```python
from build123d import *

# Parameters (mm, degrees)
SKETCH_1_W          = 56.21
SKETCH_1_H          = 40.43
EXTRUDE_1_DEPTH     = 1.5
SKETCH_2_W          = 54.71
SKETCH_2_H          = 1.5
EXTRUDE_2_DEPTH     = 3.5
SKETCH_3_W          = 1.5
SKETCH_3_H          = 8
SKETCH_3_H_2        = 18
EXTRUDE_3_DEPTH     = 3.5
SKETCH_4_W          = 2.2
SKETCH_4_H          = 1.8
EXTRUDE_4_DEPTH     = 3.5
SKETCH_5_W          = 2
SKETCH_5_H          = 1.8
EXTRUDE_5_DEPTH     = 3.5
EXTRUDE_9_DEPTH     = 7.5
SKETCH_9_R          = 0.8
CUT_EXTRUDE_1_DEPTH = 7.5
SKETCH_11_W         = 10
SKETCH_11_H         = 4
CUT_EXTRUDE_2_DEPTH = 7.5
CUT_EXTRUDE_3_DEPTH = 15


with BuildPart() as part:
    # 草图1 → 凸台-拉伸1 (new body)
    with BuildSketch(Plane(origin=(0, 0, 0), x_dir=(1, 0, 0), z_dir=(0, 1, 0))):
        with Locations((-10.770778443, 1.999730539)):
            Rectangle(SKETCH_1_W, SKETCH_1_H)
    extrude(amount=EXTRUDE_1_DEPTH)

    # 草图2 → 凸台-拉伸2 (add)
    with BuildSketch(Plane(origin=(0, 1.5, 0), x_dir=(1, 0, 0), z_dir=(0, 1, 0))):
        Polygon((-37.375778443, 22.214730539), (-38.875778443, 22.214730539), (-38.875778443, -18.215269461), (-37.375778443, -18.215269461), (-37.375778443, -16.715269461), (-37.375778443, 20.714730539), align=None)
        with Locations((-10.020778443, 21.464730539)):
            Rectangle(SKETCH_2_W, SKETCH_2_H)
        with Locations((-10.020778443, -17.465269461)):
            Rectangle(SKETCH_2_W, SKETCH_2_H)
    extrude(amount=EXTRUDE_2_DEPTH)

    # 草图3 → 凸台-拉伸3 (add)
    with BuildSketch(Plane(origin=(0, 1.5, 0), x_dir=(1, 0, 0), z_dir=(0, 1, 0))):
        with Locations((16.584221557, -12.715269461)):
            Rectangle(SKETCH_3_W, SKETCH_3_H)
        with Locations((16.584221557, 11.714730539)):
            Rectangle(SKETCH_3_W, SKETCH_3_H_2)
    extrude(amount=EXTRUDE_3_DEPTH)

    # 草图4 → 凸台-拉伸4 (add)
    with BuildSketch(Plane(origin=(0, 1.5, 0), x_dir=(1, 0, 0), z_dir=(0, 1, 0))):
        with Locations((12.934221557, 19.814730539)):
            Rectangle(SKETCH_4_W, SKETCH_4_H)
        Polygon((15.834221557, 16.714730539), (15.834221557, 20.714730539), (14.034221557, 20.714730539), (14.034221557, 18.914730539), (14.034221557, 16.714730539), align=None)
        Polygon((14.034221557, -16.715269461), (15.834221557, -16.715269461), (15.834221557, -12.715269461), (14.034221557, -12.715269461), (14.034221557, -14.915269461), align=None)
        with Locations((12.934221557, -15.815269461)):
            Rectangle(SKETCH_4_W, SKETCH_4_H)
    extrude(amount=EXTRUDE_4_DEPTH)

    # 草图5 → 凸台-拉伸5 (add)
    with BuildSketch(Plane(origin=(0, 1.5, 0), x_dir=(1, 0, 0), z_dir=(0, 1, 0))):
        with Locations((-36.375778443, 19.814730539)):
            Rectangle(SKETCH_5_W, SKETCH_5_H)
        with Locations((-36.375778443, -15.815269461)):
            Rectangle(SKETCH_5_W, SKETCH_5_H)
    extrude(amount=EXTRUDE_5_DEPTH)

    # 草图8 → 凸台-拉伸9 (add)
    with BuildSketch(Plane(origin=(0, 5, 0), x_dir=(1, 0, 0), z_dir=(0, 1, 0))):
        Polygon((17.334221557, -14.915269461), (14.034221557, -14.915269461), (11.834221557, -14.915269461), (11.834221557, -16.715269461), (-35.375778443, -16.715269461), (-35.375778443, -14.915269461), (-37.375778443, -14.915269461), (-37.375778443, 18.914730539), (-35.375778443, 18.914730539), (-35.375778443, 20.714730539), (11.834221557, 20.714730539), (11.834221557, 18.914730539), (14.034221557, 18.914730539), (17.334221557, 18.914730539), (17.334221557, 22.214730539), (-38.875778443, 22.214730539), (-38.875778443, -18.215269461), (17.334221557, -18.215269461), align=None)
    extrude(amount=EXTRUDE_9_DEPTH)

    # 草图9 → 切除-拉伸1 (cut)
    with BuildSketch(Plane(origin=(0, 12.5, 0), x_dir=(1, 0, 0), z_dir=(0, 1, 0))):
        with Locations(Location((15.684221557, 20.564730539, 0), (0, 0, 270))):
            Circle(SKETCH_9_R)
        with Locations(Location((15.684221557, -16.565269461, 0), (0, 0, 270))):
            Circle(SKETCH_9_R)
        with Locations(Location((-37.225778443, 20.564730539, 0), (0, 0, 270))):
            Circle(SKETCH_9_R)
        with Locations(Location((-37.225778443, -16.565269461, 0), (0, 0, 270))):
            Circle(SKETCH_9_R)
    extrude(amount=-CUT_EXTRUDE_1_DEPTH, mode=Mode.SUBTRACT)

    # 草图11 → 切除-拉伸2 (cut)
    with BuildSketch(Plane(origin=(-37.375778443, 0, 0), x_dir=(0, 0, -1), z_dir=(1, 0, 0))):
        with Locations((6.999730539, 3.5)):
            Rectangle(SKETCH_11_W, SKETCH_11_H)
        with Locations((-3.000269461, 3.5)):
            Rectangle(SKETCH_11_W, SKETCH_11_H)
    extrude(amount=-CUT_EXTRUDE_2_DEPTH, mode=Mode.SUBTRACT)

    # 草图14 → 切除-拉伸3 (cut)
    with BuildSketch(Plane(origin=(0, 12.5, 0), x_dir=(1, 0, 0), z_dir=(0, 1, 0))):
        with BuildLine():
            Line((-38.875778443, 22.214730539), (-38.875778443, 21.130415964))
            ThreePointArc((-38.875778443, 21.130415964), (-38.558190057, 21.897142153), (-37.791463868, 22.214730539))
            Line((-37.791463868, 22.214730539), (-38.875778443, 22.214730539))
        make_face()
        with BuildLine():
            ThreePointArc((-37.791463868, -18.215269461), (-38.558190057, -17.897681075), (-38.875778443, -17.130954886))
            Line((-38.875778443, -17.130954886), (-38.875778443, -18.215269461))
            Line((-38.875778443, -18.215269461), (-37.791463868, -18.215269461))
        make_face()
        with BuildLine():
            ThreePointArc((17.334221557, -17.130954886), (17.016633171, -17.897681075), (16.249906982, -18.215269461))
            Line((16.249906982, -18.215269461), (17.334221557, -18.215269461))
            Line((17.334221557, -18.215269461), (17.334221557, -17.130954886))
        make_face()
        with BuildLine():
            Line((17.334221557, 22.214730539), (16.249906982, 22.214730539))
            ThreePointArc((16.249906982, 22.214730539), (17.016633171, 21.897142153), (17.334221557, 21.130415964))
            Line((17.334221557, 21.130415964), (17.334221557, 22.214730539))
        make_face()
    extrude(amount=-CUT_EXTRUDE_3_DEPTH, mode=Mode.SUBTRACT)


solid = part.part
```
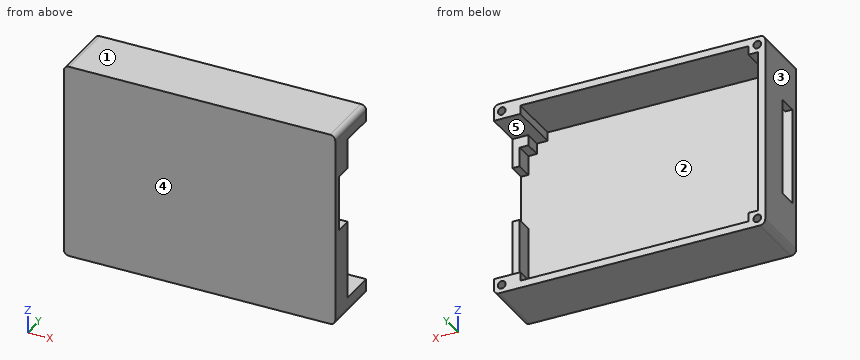
Geometry check sheet. Reference: the model listing, model coordinates, mm. Face numbers are marked on the shaded views. A direction names the side the tool comes from. Give positions to 0.01 mm unless a question says otherwise; leave off trailing zeros. Write each loop counter-clockwise with the first axis right and the second up, starting at its lowest first coordinate (ties: lowest second). Pieces come first, ordered by that corner, then holes. Notation, with made-up numbers: (-1, 75.5) - (46, 75.5) arc R20 cw to (46, 88.5) - close; hole circle Ø3 at (75.5, -15). An arc over 180 degrees is marked (long way). Use a Markdown table: item, result.
Q1. Go/stop test with flat-tipped pins: P1, Ø4, axis at x = -15.5, z = -10.5, coming from the +Y side; P2, Ø1.4, axis at x = 15.68, z = -20.56, coming from the +Y side. Record where each tip stops, or that it passes through.
Computed:
| item | result |
|---|---|
| P1 | stops at y = 1.5 |
| P2 | stops at y = 5 |
Q2. Draft check along X on the marked faces 1, 2 and 3. Enter one of: pulls with the +X half, pulls with the -X half, needs draft (parallel to the pull), parting line crosses it, or undercut.
Computed:
| item | result |
|---|---|
| face 1 | needs draft |
| face 2 | undercut |
| face 3 | pulls with the -X half |
Q3. Section check C-C, the plane x = 5. Enter the section's corners in (y, z), then the cut area to 3 significant figures.
Computed:
| item | result |
|---|---|
| outline | (0, -22.21) - (12.5, -22.21) - (12.5, -20.71) - (1.5, -20.71) - (1.5, 16.72) - (12.5, 16.72) - (12.5, 18.22) - (0, 18.22) - close |
| area | 93.6 mm² |
Q4. Section check D-D, the plane y = 7. Enter the section's corners in (x, z).
Computed:
| item | result |
|---|---|
| outline | (-38.88, -21.13) arc R1.08 ccw to (-37.79, -22.21) - (16.25, -22.21) arc R1.08 ccw to (17.33, -21.13) - (17.33, -18.91) - (11.83, -18.91) - (11.83, -20.71) - (-35.38, -20.71) - (-35.38, -18.91) - (-37.38, -18.91) - (-37.38, 14.92) - (-35.38, 14.92) - (-35.38, 16.72) - (11.83, 16.72) - (11.83, 14.92) - (17.33, 14.92) - (17.33, 17.13) arc R1.08 ccw to (16.25, 18.22) - (-37.79, 18.22) arc R1.08 ccw to (-38.88, 17.13) - close; hole circle Ø1.6 at (-37.23, -20.56); hole circle Ø1.6 at (-37.23, 16.57); hole circle Ø1.6 at (15.68, -20.56); hole circle Ø1.6 at (15.68, 16.57) |
Q5. Section check A-A, the plane z = -9. Enter the section's corners in (x, y).
Computed:
| item | result |
|---|---|
| outline | (-38.88, 0) - (17.33, 0) - (17.33, 5) - (15.83, 5) - (15.83, 1.5) - (-38.88, 1.5) - close; (-38.88, 5.5) - (-37.38, 5.5) - (-37.38, 12.5) - (-38.88, 12.5) - close |
Q6. Thickness scan on L1, parallel to Z at x = -3.5, y = 4.75; L2, parallel to X at y = 3.75, z = 16.5; L3, parallel to X at y = 4.5, z = 12.5. Record the ranges inside material, lowest first. Write a range as [from, to].
Computed:
| item | result |
|---|---|
| L1 | z = [-22.21, -20.71], [16.72, 18.22] |
| L2 | x = [-38.88, -35.38], [11.83, 17.33] |
| L3 | x = [-38.88, -37.38], [15.83, 17.33] |
Q7. Set-up check for the marked faces 4 and 5: record each of +Z, -Z, +X, -X, +Y, -Y from which the full face is reachable in a straight line by a thin tool's end or side.
Computed:
| item | result |
|---|---|
| face 4 | +Z, -Z, +X, -X, -Y |
| face 5 | +Y |
